```python
from build123d import *

# Parameters (mm, degrees)
SKETCH2_W                       = 70
SKETCH2_H                       = 100
BOSS_EXTRUDE1_DEPTH             = 2.5
SKETCH3_R                       = 3.5
SKETCH3_R_2                     = 1.5
BOSS_EXTRUDE2_DEPTH             = 5
BOSS_EXTRUDE2_DIRECTION_2_REACH = 150.961


with BuildPart() as part:
    # Sketch2 → Boss-Extrude1 (new body)
    with BuildSketch(Plane(origin=(0, 0, 0), x_dir=(1, 0, 0), z_dir=(0, 1, 0))):
        with Locations((74, 51.5)):
            Rectangle(SKETCH2_W, SKETCH2_H)
    extrude(amount=BOSS_EXTRUDE1_DEPTH)

    # Sketch3 → Boss-Extrude2 (add)
    # profile 1 of 5: a face of its own
    with BuildSketch(Plane(origin=(0, 2.5, 0), x_dir=(1, 0, 0), z_dir=(0, 1, 0))):
        with Locations(Location((41.25, 3.75, 0), (0, 0, 270))):
            Circle(SKETCH3_R)
        with Locations(Location((41.25, 3.75, 0), (0, 0, 270))):
            Circle(SKETCH3_R_2, mode=Mode.SUBTRACT)
    # profile 2 of 5: a face of its own
    with BuildSketch(Plane(origin=(0, 2.5, 0), x_dir=(1, 0, 0), z_dir=(0, 1, 0))):
        with Locations(Location((106, 19.5, 0), (0, 0, 270))):
            Circle(SKETCH3_R)
        with Locations(Location((106, 19.5, 0), (0, 0, 270))):
            Circle(SKETCH3_R_2, mode=Mode.SUBTRACT)
    # profile 3 of 5: a face of its own
    with BuildSketch(Plane(origin=(0, 2.5, 0), x_dir=(1, 0, 0), z_dir=(0, 1, 0))):
        with Locations(Location((106, 81.5, 0), (0, 0, 270))):
            Circle(SKETCH3_R)
        with Locations(Location((106, 81.5, 0), (0, 0, 270))):
            Circle(SKETCH3_R_2, mode=Mode.SUBTRACT)
    # profile 4 of 5: a face of its own
    with BuildSketch(Plane(origin=(0, 2.5, 0), x_dir=(1, 0, 0), z_dir=(0, 1, 0))):
        with Locations(Location((68.3, 67.9, 0), (0, 0, 270))):
            Circle(SKETCH3_R)
        with Locations(Location((68.3, 67.9, 0), (0, 0, 270))):
            Circle(SKETCH3_R_2, mode=Mode.SUBTRACT)
    # profile 5 of 5: a face of its own
    with BuildSketch(Plane(origin=(0, 2.5, 0), x_dir=(1, 0, 0), z_dir=(0, 1, 0))):
        with Locations(Location((71.1, 99.7, 0), (0, 0, 270))):
            Circle(SKETCH3_R)
        with Locations(Location((71.1, 99.7, 0), (0, 0, 270))):
            Circle(SKETCH3_R_2, mode=Mode.SUBTRACT)
    extrude(amount=BOSS_EXTRUDE2_DEPTH)

    # Boss-Extrude2 direction 2: up to this face of the body (flat: up to its plane)
    boss_extrude2_direction_2_end = Plane(part.part.faces().sort_by_distance((74, 0, -51.5))[0])
    # Sketch3 → Boss-Extrude2 direction 2 (add, up to the picked face)
    with BuildSketch(Plane(origin=(0, 2.5, 0), x_dir=(1, 0, 0), z_dir=(0, 1, 0)), mode=Mode.PRIVATE) as boss_extrude2_direction_2_sk1:
        with Locations(Location((41.25, 3.75, 0), (0, 0, 270))):
            Circle(SKETCH3_R)
        with Locations(Location((41.25, 3.75, 0), (0, 0, 270))):
            Circle(SKETCH3_R_2, mode=Mode.SUBTRACT)
    boss_extrude2_direction_2_tool1 = split(extrude(boss_extrude2_direction_2_sk1.sketch, amount=-BOSS_EXTRUDE2_DIRECTION_2_REACH, mode=Mode.PRIVATE), bisect_by=boss_extrude2_direction_2_end, keep=Keep.BOTH, mode=Mode.PRIVATE)
    # Sketch3 → Boss-Extrude2 direction 2 (add, up to the picked face)
    with BuildSketch(Plane(origin=(0, 2.5, 0), x_dir=(1, 0, 0), z_dir=(0, 1, 0)), mode=Mode.PRIVATE) as boss_extrude2_direction_2_sk2:
        with Locations(Location((106, 19.5, 0), (0, 0, 270))):
            Circle(SKETCH3_R)
        with Locations(Location((106, 19.5, 0), (0, 0, 270))):
            Circle(SKETCH3_R_2, mode=Mode.SUBTRACT)
    boss_extrude2_direction_2_tool2 = split(extrude(boss_extrude2_direction_2_sk2.sketch, amount=-BOSS_EXTRUDE2_DIRECTION_2_REACH, mode=Mode.PRIVATE), bisect_by=boss_extrude2_direction_2_end, keep=Keep.BOTH, mode=Mode.PRIVATE)
    # Sketch3 → Boss-Extrude2 direction 2 (add, up to the picked face)
    with BuildSketch(Plane(origin=(0, 2.5, 0), x_dir=(1, 0, 0), z_dir=(0, 1, 0)), mode=Mode.PRIVATE) as boss_extrude2_direction_2_sk3:
        with Locations(Location((106, 81.5, 0), (0, 0, 270))):
            Circle(SKETCH3_R)
        with Locations(Location((106, 81.5, 0), (0, 0, 270))):
            Circle(SKETCH3_R_2, mode=Mode.SUBTRACT)
    boss_extrude2_direction_2_tool3 = split(extrude(boss_extrude2_direction_2_sk3.sketch, amount=-BOSS_EXTRUDE2_DIRECTION_2_REACH, mode=Mode.PRIVATE), bisect_by=boss_extrude2_direction_2_end, keep=Keep.BOTH, mode=Mode.PRIVATE)
    # Sketch3 → Boss-Extrude2 direction 2 (add, up to the picked face)
    with BuildSketch(Plane(origin=(0, 2.5, 0), x_dir=(1, 0, 0), z_dir=(0, 1, 0)), mode=Mode.PRIVATE) as boss_extrude2_direction_2_sk4:
        with Locations(Location((68.3, 67.9, 0), (0, 0, 270))):
            Circle(SKETCH3_R)
        with Locations(Location((68.3, 67.9, 0), (0, 0, 270))):
            Circle(SKETCH3_R_2, mode=Mode.SUBTRACT)
    boss_extrude2_direction_2_tool4 = split(extrude(boss_extrude2_direction_2_sk4.sketch, amount=-BOSS_EXTRUDE2_DIRECTION_2_REACH, mode=Mode.PRIVATE), bisect_by=boss_extrude2_direction_2_end, keep=Keep.BOTH, mode=Mode.PRIVATE)
    # Sketch3 → Boss-Extrude2 direction 2 (add, up to the picked face)
    with BuildSketch(Plane(origin=(0, 2.5, 0), x_dir=(1, 0, 0), z_dir=(0, 1, 0)), mode=Mode.PRIVATE) as boss_extrude2_direction_2_sk5:
        with Locations(Location((71.1, 99.7, 0), (0, 0, 270))):
            Circle(SKETCH3_R)
        with Locations(Location((71.1, 99.7, 0), (0, 0, 270))):
            Circle(SKETCH3_R_2, mode=Mode.SUBTRACT)
    boss_extrude2_direction_2_tool5 = split(extrude(boss_extrude2_direction_2_sk5.sketch, amount=-BOSS_EXTRUDE2_DIRECTION_2_REACH, mode=Mode.PRIVATE), bisect_by=boss_extrude2_direction_2_end, keep=Keep.BOTH, mode=Mode.PRIVATE)
    add(boss_extrude2_direction_2_tool1.solids().sort_by(Axis((41.25, 2.5, -7.151005), (0, -1, 0)))[0])
    add(boss_extrude2_direction_2_tool2.solids().sort_by(Axis((106, 2.5, -22.901005), (0, -1, 0)))[0])
    add(boss_extrude2_direction_2_tool3.solids().sort_by(Axis((106, 2.5, -84.901005), (0, -1, 0)))[0])
    add(boss_extrude2_direction_2_tool4.solids().sort_by(Axis((68.3, 2.5, -71.301005), (0, -1, 0)))[0])
    add(boss_extrude2_direction_2_tool5.solids().sort_by(Axis((71.1, 2.5, -103.101005), (0, -1, 0)))[0])


solid = part.part
```
Verification items for the finished model (mm, model axes). A direction names the side the tool comes from. Give positions to 0.01 mm unless a question says otherwise; leave off trailing zeros. Order: outer loops, then holes, each group sorted by start corner. A loop starts at its lowest first (then second) coordinate and runs counter-clockwise, first axis right, second up. Notation, with made-up numbers: (24.25, 53) -> (35.25, 53) arc R19 ccw to (35.25, 86) -> close; hole circle Ø5 at (49.5, 35). An arc over 180 degrees is marked (long way). One line per item, written item: value.
(1) Scan lines: line 1 along Z through (x, y) = (106, 4); line 2 along X through (y, z) = (5.6, -67.9); line 3 along X through (y, z) = (6.25, -3.75). Record each from-to range of solid material in increasing order. Write a range as [from, to].
Final values:
line 1: [-85, -83], [-80, -78], [-23, -21], [-18, -16]
line 2: [64.8, 66.8], [69.8, 71.8]
line 3: [37.75, 39.75], [42.75, 44.75]
(2) Gauge pin test, flat ends, axial feed: pin 1 (1.5 mm diameter, centred on x = 93.5, z = -24.5, fed in from +Y); pin 2 (3.5 mm diameter, centred on x = 71.5, z = -99.5, fed in from +Y); pin 3 (1.2 mm diameter, centred on y = 1.5, z = -72.5, fed in from -X); pin 4 (0.8 mm diameter, centred on x = 84, y = 1.5, fed in from +Z). Record the tip position at first contact, or that the pin passes through.
Final values:
pin 1: y = 2.5
pin 2: y = 7.5
pin 3: x = 39
pin 4: z = -1.5
(3) Sectioned sample at C-C on x = 94.5. Record the cut outline in (y, z).
Final values:
outline: (0, -101.5) -> (2.5, -101.5) -> (2.5, -1.5) -> (0, -1.5) -> close
(4) Sectioned sample at D-D on z = -19.5. Record the cut outline in (x, y).
Final values:
outline: (39, 0) -> (109.5, 0) -> (109.5, 7.5) -> (107.5, 7.5) -> (107.5, 2.5) -> (104.5, 2.5) -> (104.5, 7.5) -> (102.5, 7.5) -> (102.5, 2.5) -> (39, 2.5) -> close
(5) Draft check along X on faces 6 (the face through (106, 2.5, -20)), 7 (the face through (39, 1, -53)), 8 (the face through (109, 1, -50)). Enter one of: pulls with the +X half, pulls with the -X half, needs draft (parallel to the pull), parting line crosses it, or undercut.
Final values:
face 6: undercut
face 7: pulls with the -X half
face 8: pulls with the +X half
(6) Sectioned sample at B-B on z = -67.9. Record the cut outline in (x, y).
Final values:
outline: (39, 0) -> (109, 0) -> (109, 2.5) -> (71.8, 2.5) -> (71.8, 7.5) -> (69.8, 7.5) -> (69.8, 2.5) -> (66.8, 2.5) -> (66.8, 7.5) -> (64.8, 7.5) -> (64.8, 2.5) -> (39, 2.5) -> close
(7) Sectioned sample at A-A on y = 1.25. Record the cut outline in (x, z).
Final values:
outline: (39, -101.5) -> (68.1, -101.5) arc R3.5 ccw to (74.1, -101.5) -> (109, -101.5) -> (109, -83.3) arc R3.5 ccw to (109, -79.7) -> (109, -21.3) arc R3.5 ccw to (109, -17.7) -> (109, -1.5) -> (43.93, -1.5) arc R3.5 ccw (long way) to (39, -6.43) -> close
(8) Tool access check on faces 1 (the face through (109, 1, -9)), 2 (the face through (41, 2.5, -4)), 3 (the face through (73, 0, -51)), 4 (the face through (109, 1, -92)), 5 (the face through (41, 7.5, -2)). Record the directions out of +Z, -Z, +X, -X, +Y, -Y that give a thin tool (end or side, any length) a straight path to the whole face; none if there is none.
Final values:
face 1: +Z, +X, +Y, -Y
face 2: +Y
face 3: +Z, -Z, +X, -X, -Y
face 4: -Z, +X, +Y, -Y
face 5: +Z, -Z, +X, -X, +Y
